from build123d import *

# Parameters (mm, degrees)
F1_DEPTH = 15
F2_DEPTH = 15
F3_DEPTH = 11
F4_DEPTH = 3.1
F6_DEPTH = 3


with BuildPart() as f1:
    # F0 (on Top) → F1 (new body)
    with BuildSketch(Plane.XY):
        with BuildLine():
            ThreePointArc((9.8868599666, 1.5), (7.3340931671, 6.7978730068), (2.2448979592, 9.744764397))
            ThreePointArc((2.2448979592, 9.744764397), (-10, 0), (2.2448979592, -9.744764397))
            ThreePointArc((2.2448979592, -9.744764397), (7.3340931671, -6.7978730068), (9.8868599666, -1.5))
            Line((9.8868599666, -1.5), (5.8094750193, -1.5))
            ThreePointArc((5.8094750193, -1.5), (-6, 0), (5.8094750193, 1.5))
            Line((5.8094750193, 1.5), (9.8868599666, 1.5))
        make_face()
        with BuildLine():
            ThreePointArc((10, 0), (9.971674876, 0.7521304187), (9.8868599666, 1.5))
            Line((9.8868599666, 1.5), (5.8094750193, 1.5))
            ThreePointArc((5.8094750193, 1.5), (5.9521781776, 0.7560257549), (6, 0))
            ThreePointArc((6, 0), (5.9521781776, -0.7560257549), (5.8094750193, -1.5))
            Line((5.8094750193, -1.5), (9.8868599666, -1.5))
            ThreePointArc((9.8868599666, -1.5), (9.971674876, -0.7521304187), (10, 0))
        make_face()
    extrude(amount=F1_DEPTH)

    # F0 (on Top) → F2 (join)
    with BuildSketch(Plane.XY):
        with BuildLine():
            Line((20.2573593129, 1.5), (9.8868599666, 1.5))
            ThreePointArc((9.8868599666, 1.5), (9.971674876, 0.7521304187), (10, 0))
            ThreePointArc((10, 0), (9.971674876, -0.7521304187), (9.8868599666, -1.5))
            Line((9.8868599666, -1.5), (20.2573593129, -1.5))
            ThreePointArc((20.2573593129, -1.5), (20, 0), (20.2573593129, 1.5))
        make_face()
        with BuildLine():
            Line((22.5, 1.5), (20.2573593129, 1.5))
            ThreePointArc((20.2573593129, 1.5), (20, 0), (20.2573593129, -1.5))
            Line((20.2573593129, -1.5), (22.5, -1.5))
            ThreePointArc((22.5, -1.5), (22, 0), (22.5, 1.5))
        make_face()
    extrude(amount=F2_DEPTH)

    # F0 (on Top) → F3 (join)
    with BuildSketch(Plane.XY):
        with BuildLine():
            ThreePointArc((29, 0), (28.021073584, 2.8021493208), (25.5102040816, 4.3851439786))
            ThreePointArc((25.5102040816, 4.3851439786), (22.3336261757, 3.9442140476), (20.2573593129, 1.5))
            Line((20.2573593129, 1.5), (22.5, 1.5))
            ThreePointArc((22.5, 1.5), (25.290569415, 2.3717082451), (27, 0))
            ThreePointArc((27, 0), (25.290569415, -2.3717082451), (22.5, -1.5))
            Line((22.5, -1.5), (20.2573593129, -1.5))
            ThreePointArc((20.2573593129, -1.5), (22.3336261757, -3.9442140476), (25.5102040816, -4.3851439786))
            ThreePointArc((25.5102040816, -4.3851439786), (28.021073584, -2.8021493208), (29, 0))
        make_face()
    extrude(amount=F3_DEPTH)

    # F0 (on Top) → F4 (join)
    with BuildSketch(Plane.XY):
        with BuildLine():
            ThreePointArc((9.8868599666, -1.5), (7.3340931671, -6.7978730068), (2.2448979592, -9.744764397))
            Line((2.2448979592, -9.744764397), (25.5102040816, -4.3851439786))
            ThreePointArc((25.5102040816, -4.3851439786), (22.3336261757, -3.9442140476), (20.2573593129, -1.5))
            Line((20.2573593129, -1.5), (9.8868599666, -1.5))
        make_face()
        with BuildLine():
            Line((25.5102040816, 4.3851439786), (2.2448979592, 9.744764397))
            ThreePointArc((2.2448979592, 9.744764397), (7.3340931671, 6.7978730068), (9.8868599666, 1.5))
            Line((9.8868599666, 1.5), (20.2573593129, 1.5))
            ThreePointArc((20.2573593129, 1.5), (22.3336261757, 3.9442140476), (25.5102040816, 4.3851439786))
        make_face()
    extrude(amount=F4_DEPTH)

    # F5 (on face) → F6 (cut, through all)
    with BuildSketch(Plane.XZ.offset(1.5)):
        Polygon((22.5, 15), (9.8868599666, 15), (20.2573593129, 11), (22.5, 11), align=None)
    extrude(amount=-F6_DEPTH, mode=Mode.SUBTRACT)


solid = f1.part
Could you check a few things on this model? Use its own coordinates, in mm. A direction names the side the tool comes from. Give positions to 0.01 mm unless a question says otherwise; leave off trailing zeros. Order: outer loops, then holes, each group sorted by start corner. A loop starts at its lowest first (then second) coordinate and runs counter-clockwise, first axis right, second up. Notation, with made-up numbers: (52, 62.25) -> (80, 62.25) arc R26 ccw to (80, 97.25) -> close; hole circle Ø4 at (-21.5, -1.5). An arc over 180 degrees is marked (long way). Answer in a Markdown table with one row per item. Add a question column.
Item 1: Imagine slicing it at A-A (x = 0). List the corners of the cut face in (y, z) for me, and give its area (3 significant figures).
Item 2: For faces 5 (the flat face through (22.6, -1.9, 11)), 6 (the flat face through (14, 5, 3.1)), 7 (the flat face through (14, -5, 3.1)), which set-ups out of +Z, -Z, +X, -X, +Y, -Y let a thin tool reach every point of the face, with its end or its side?
Item 3: I'm going to push flat-ended pins straight in: P1, Ø8, axis at y = -7.5, z = 5.5, coming from the +X side; P2, Ø3, axis at x = 13.5, z = 8, coming from the +Y side; P3, Ø8, axis at y = 4.5, z = 13.5, coming from the -X side. Where does each tip first touch, or does it pass through?
Item 4: Imagine slicing it at B-B (z = 10). List the corners of the cut face in (x, y) for me.
Item 5: Please list where these lines run through material, in increasing order: probe 1 along Y at (x, z) = (0, 9.5); probe 2 along Z at (x, y) = (8, -6.25); probe 3 along X at (y, z) = (-2, 10.25).
Item 6: Imagine slicing it at C-C (y = 1). List the corners of the cut face in (x, z) for me, and give its area (3 significant figures).
Item 7: We'd pull the mould along X, two halves only. Please class faces 1 (the flat face through (9, 0, 0)), 2 (the flat face through (13.715, -7.102, 1.528)), 3 (the flat face through (15, -1.5, 8)), 4 (the flat face through (15, 1.5, 8)): pulls with the +X half, pulls with the -X half, needs draft (parallel to the pull), parting line crosses it, or undercut.
Item 8: Imagine slicing it at D-D (x = 13). List the corners of the cut face in (y, z) for me.
Result:
| question | item | result |
|---|---|---|
| 1 | outline | (-10, 0) -> (-6, 0) -> (-6, 15) -> (-10, 15) -> close; (6, 0) -> (10, 0) -> (10, 15) -> (6, 15) -> close |
| 1 | area | 120 mm2 |
| 2 | face 5 | +Z, +X, +Y, -Y |
| 2 | face 6 | +Z, +Y |
| 2 | face 7 | +Z, -Y |
| 3 | P1 | x = 27.33 |
| 3 | P2 | y = 1.5 |
| 3 | P3 | x = -9.99 |
| 4 | outline | (9.89, -1.5) -> (20.26, -1.5) arc R4.5 ccw (long way) to (20.26, 1.5) -> (9.89, 1.5) arc R10 ccw (long way) to start; hole circle Ø12 at (0, 0); hole circle Ø5 at (24.5, 0) |
| 5 | probe 1 | -10 to -6, 6 to 10 |
| 5 | probe 2 | 0 to 3.1 |
| 5 | probe 3 | -9.8 to -5.66, 5.66 to 9.8, 20.47 to 23, 26 to 28.53 |
| 6 | outline | (-9.95, 0) -> (-5.92, 0) -> (-5.92, 15) -> (-9.95, 15) -> close; (5.92, 0) -> (22.21, 0) -> (22.21, 11) -> (20.26, 11) -> (9.89, 15) -> (5.92, 15) -> close; (26.79, 0) -> (28.89, 0) -> (28.89, 11) -> (26.79, 11) -> close |
| 6 | area | 299 mm2 |
| 7 | face 1 | needs draft |
| 7 | face 2 | pulls with the +X half |
| 7 | face 3 | undercut |
| 7 | face 4 | undercut |
| 8 | outline | (-7.27, 0) -> (7.27, 0) -> (7.27, 3.1) -> (1.5, 3.1) -> (1.5, 13.8) -> (-1.5, 13.8) -> (-1.5, 3.1) -> (-7.27, 3.1) -> close |
